```python
from build123d import *

# Parameters (mm, degrees)
ESBO_O1_R                                  = 3
RESSALTO_EXTRUS_O1_DEPTH                   = 40
BROCA_DE_ROSQUEAR_PARA_HELICOIDE_M31_D     = 3.15
BROCA_DE_ROSQUEAR_PARA_HELICOIDE_M31_DEPTH = 4
BROCA_DE_ROSQUEAR_PARA_HELICOIDE_M31_TIP   = 0.946355475
BROCA_DE_ROSQUEAR_PARA_HELICOIDE_M32_D     = 3.15
BROCA_DE_ROSQUEAR_PARA_HELICOIDE_M32_DEPTH = 4
BROCA_DE_ROSQUEAR_PARA_HELICOIDE_M32_TIP   = 0.946355475


with BuildPart() as part:
    # Esboço1 → Ressalto-extrusão1 (new body)
    with BuildSketch(Plane.XY):
        Circle(ESBO_O1_R)
    extrude(amount=RESSALTO_EXTRUS_O1_DEPTH)

    # Broca de rosquear para helicoide M31
    with Locations(Plane(origin=(0, 0, 0), x_dir=(-1, 0, 0), z_dir=(0, 0, -1))):
        with Locations((0, 0)):
            Hole(BROCA_DE_ROSQUEAR_PARA_HELICOIDE_M31_D / 2, depth=BROCA_DE_ROSQUEAR_PARA_HELICOIDE_M31_DEPTH)
            with Locations((0, 0, -(BROCA_DE_ROSQUEAR_PARA_HELICOIDE_M31_DEPTH + BROCA_DE_ROSQUEAR_PARA_HELICOIDE_M31_TIP / 2))):  # 118° drill point
                Cone(0, BROCA_DE_ROSQUEAR_PARA_HELICOIDE_M31_D / 2, BROCA_DE_ROSQUEAR_PARA_HELICOIDE_M31_TIP, mode=Mode.SUBTRACT)

    # Broca de rosquear para helicoide M32
    with Locations(Plane.XY.offset(40)):
        with Locations((0, 0)):
            Hole(BROCA_DE_ROSQUEAR_PARA_HELICOIDE_M32_D / 2, depth=BROCA_DE_ROSQUEAR_PARA_HELICOIDE_M32_DEPTH)
            with Locations((0, 0, -(BROCA_DE_ROSQUEAR_PARA_HELICOIDE_M32_DEPTH + BROCA_DE_ROSQUEAR_PARA_HELICOIDE_M32_TIP / 2))):  # 118° drill point
                Cone(0, BROCA_DE_ROSQUEAR_PARA_HELICOIDE_M32_D / 2, BROCA_DE_ROSQUEAR_PARA_HELICOIDE_M32_TIP, mode=Mode.SUBTRACT)


solid = part.part
```
Model file for the job. Use its own axes, mm. A direction names the side the tool comes from. Round coordinates to 2 decimals unless told otherwise and drop trailing zeros. Write each loop counter-clockwise with the first axis right and the second up, starting at its lowest first coordinate (ties: lowest second). Pieces come first, ordered by that corner, then holes. Notation, with made-up numbers: (79.5, -21) - (116.5, -21) arc R6 ccw to (116.5, -16) - close; hole circle Ø6 at (39.5, 66). An arc over 180 degrees is marked (long way). Use CSV: the item, a comma, the result in double quotes. Start each with the question number.
Item 1: Two-plate mould, pull along Y, no slides. Class faces 1 (the face through (-1.25, -0.96, 2.03)), 2 (the face through (1.3, -1.3, 0)), 3 (the face through (-3, 0, 20)): released by +Y, released by -Y, zero draft, split by the parting line, or undercut.
Item 2: Pin check, flat tips, straight feed: P1, Ø1.9, axis at x = 0, y = 0, coming from the -Z side; P2, Ø3, axis at x = 0, y = 0, coming from the +Z side; P3, Ø3, axis at y = -2.5, z = 34, coming from the +X side. Stop position of each tip, or through.
Item 3: Band-saw the part on A-A (z = 7). Write the cut outline in (x, y), and give its area (3 significant figures).
Item 4: Band-saw the part on B-B (y = -2.1). Write the cut outline in (x, z).
Item 5: Drill centre lines: L1, parallel to Y at x = 0, z = 1.75 (3 decimals); L2, parallel to Y at x = 0.7, z = 2.5; L3, parallel to X at y = 0.2, z = 32.5. Where is each one in solid material? Low to high. Write a range as [from, to].
Item 6: Tool access for faces 4 (the face through (1.25, -0.96, 37.97)), 5 (the face through (1.3, -1.3, 40)): list every direction of +Z, -Z, +X, -X, +Y, -Y with a clear straight run to the whole face (end or side of a thin tool).
Checked values:
1,face 1,"undercut"
1,face 2,"zero draft"
1,face 3,"split by the parting line"
2,P1,"stops at z = 4.38"
2,P2,"stops at z = 35.95"
2,P3,"stops at x = 2.83"
3,outline,"circle Ø6 at (0, 0)"
3,area,"28.3 mm²"
4,outline,"(-2.14, 0) - (2.14, 0) - (2.14, 40) - (-2.14, 40) - close"
5,L1,"y = [-3, -1.575], [1.575, 3]"
5,L2,"y = [-2.92, -1.41], [1.41, 2.92]"
5,L3,"x = [-2.99, 2.99]"
6,face 4,"+Z"
6,face 5,"+Z, +X, -X, +Y, -Y"
